Can you work these out from the model? Positions are in its coordinate system, mm. A direction names the side the tool comes from. Round coordinates to 2 decimals unless told otherwise and drop trailing zeros. Write each loop counter-clockwise with the first axis right and the second up, starting at its lowest first coordinate (ties: lowest second). Pieces come first, ordered by that corner, then holes. Notation, with made-up numbers: M 50,51.5 L 104,51.5 A23 ccw 104,79.5 Z; hole C 81,63 d4. An arc over 180 degrees is marked long. Use one line per item in the form item = value. Start each with the question number.
```python
from build123d import *

# Parameters (mm, degrees)
BOSS_EXTRUDE1_DEPTH = 35
SKETCH3_W           = 12
SKETCH3_H           = 16
CUT_EXTRUDE1_DEPTH  = 35
BOSS_EXTRUDE2_REACH = 93.924
SKETCH4_W           = 17.5
SKETCH4_H           = 17.5
CUT_EXTRUDE2_DEPTH  = 92.923881554


with BuildPart() as part:
    # Sketch2 → Boss-Extrude1 (new body)
    with BuildSketch(Plane.XY):
        Polygon((25, 25), (25, 0), (75, 0), (75, 15), (40, 15), (40, 40), (0, 40), (0, 25), align=None)
    extrude(amount=BOSS_EXTRUDE1_DEPTH)

    # Sketch3 → Cut-Extrude1 (cut)
    with BuildSketch(Plane(origin=(0, 40, 0), x_dir=(1, 0, 0), z_dir=(0, 1, 0))):
        with Locations((6, -17.5)):
            Rectangle(SKETCH3_W, SKETCH3_H)
    extrude(amount=-CUT_EXTRUDE1_DEPTH, mode=Mode.SUBTRACT)

    # Sketch4 → Boss-Extrude2 (add, up to next)
    with BuildSketch(Plane(origin=(0, 40, 0), x_dir=(1, 0, 0), z_dir=(0, 1, 0)), mode=Mode.PRIVATE) as boss_extrude2_sk1:
        with Locations((48.75, -8.75)):
            Rectangle(SKETCH4_W, SKETCH4_H)
    boss_extrude2_tool1 = extrude(boss_extrude2_sk1.sketch, amount=-BOSS_EXTRUDE2_REACH, mode=Mode.PRIVATE) - part.part
    add(boss_extrude2_tool1.solids().sort_by_distance((48.75, 40, 8.75))[0])

    # Sketch5 → Cut-Extrude2 (cut, through all)
    with BuildSketch(Plane(origin=(75, 0, 0), x_dir=(0, 0, -1), z_dir=(1, 0, 0))):
        Polygon((-26.878944817, 0), (-22.837492933, 7), (-10.920396702, 7), (-6.878944817, 0), align=None)
    extrude(amount=-CUT_EXTRUDE2_DEPTH, mode=Mode.SUBTRACT)


solid = part.part
```
1. Will these pins go through, and if not, where does the flat tip stop? pin 1 (12 mm diameter, centred on y = 30, z = 18.5, fed in from -X); pin 2 (12.5 mm diameter, centred on x = 7.5, z = 9.5, fed in from -Y); pin 3 (10 mm diameter, centred on x = 55, y = 20.5, fed in from +Z).
2. If we section it at D-D (y = 3): List the corners of the cut face in (x, z) for me.
3. Please list where these lines run through material, in increasing order: line 1 along X through (y, z) = (25.5, 16.5); line 2 along X through (y, z) = (17, 11.5); line 3 along Y through (x, z) = (29.5, 16).
4. If we mould it in two halves opening along Z, with no side actions, what happens to faces 6 (the face through (50.4, 3.5, 8.9)), 7 (the face through (49, 28, 17.5)), 8 (the face through (0, 33, 30)), 9 (the face through (50.35, 3.451, 24.887))? For each: pulls with the +Z half, pulls with the -Z half, needs draft (parallel to the pull), parting line crosses it, or undercut.
5. If we section it at C-C (x = 53.5): List the corners of the cut face in (y, z) for me.
6. Which directions (+Z, -Z, +X, -X, +Y, -Y) give clear straight access to the entire face, cutting with the end or side of a thin tool? Please do faces 1 (the face through (57.5, 28, 9)), 2 (the face through (50, 7, 17)), 3 (the face through (12, 33, 18)), 4 (the face through (40, 27, 26)), 5 (the face through (25, 13, 17)).
7. If we section it at B-B (z = 28): List the corners of the cut face in (x, y) for me, and give its area (3 significant figures).
8. If we section it at A-A (x = 5.5): List the corners of the cut face in (y, z) for me.
Model answer:
q1.pin_1 = 12
q1.pin_2 = 25
q1.pin_3 = 17.5
q2.outline = M 25,0 L 75,0 L 75,8.61 L 25,8.61 Z; M 25,25.15 L 75,25.15 L 75,35 L 25,35 Z
q3.line_1 = 12 to 57.5
q3.line_2 = 25 to 57.5
q3.line_3 = 7 to 40
q4.face_6 = undercut
q4.face_7 = pulls with the +Z half
q4.face_8 = needs draft
q4.face_9 = undercut
q5.outline = M 0,0 L 40,0 L 40,17.5 L 15,17.5 L 15,35 L 0,35 L 0,26.88 L 7,22.84 L 7,10.92 L 0,6.88 Z
q6.face_1 = +Z, -Z, +X, +Y
q6.face_2 = +X, -X, -Y
q6.face_3 = -X, +Y, -Y
q6.face_4 = +Z, +X, +Y
q6.face_5 = +Z, -Z, -X, -Y
q7.outline = M 0,25 L 25,25 L 25,0 L 75,0 L 75,15 L 40,15 L 40,40 L 0,40 Z
q7.area = 1,500 mm2
q8.outline = M 25,0 L 40,0 L 40,9.5 L 25,9.5 Z; M 25,25.5 L 40,25.5 L 40,35 L 25,35 Z
